The model under review builds one solid part; all positions refer to its coordinate system, in mm. Face numbers are marked on the shaded views. A direction names the side the tool comes from. Coordinates: 2 decimals unless noted, no trailing zeros. Order: outer loops, then holes, each group sorted by start corner. A loop starts at its lowest first (then second) coordinate and runs counter-clockwise, first axis right, second up. Notation, with made-up numbers: (86, 2.25) -> (116, 2.25) arc R12 ccw to (116, 6.25) -> close; hole circle Ø8 at (-15, 81). An arc over 180 degrees is marked (long way). Put each result on its own line as item: value.
from build123d import *

# Parameters (mm, degrees)
ESQUISSE2_W             = 60
ESQUISSE2_H             = 30
BOSS_EXTRU_1_DEPTH      = 15
ESQUISSE3_R             = 5
BOSS_EXTRU_2_DEPTH      = 6
BOSS_EXTRU_3_DEPTH      = 20
ESQUISSE5_R             = 5
ENL_V_MAT_EXTRU_1_DEPTH = 30
ESQUISSE6_W             = 3
ESQUISSE6_H             = 20
BOSS_EXTRU_4_DEPTH      = 15
CONG_2_R                = 10
CONG_3_R                = 10
CONG_4_R                = 10
CONG_5_R                = 10
ESQUISSE7_R             = 3
ENL_V_MAT_EXTRU_2_DEPTH = 27


with BuildPart() as part:
    # Esquisse2 → Boss.-Extru.1 (new body)
    with BuildSketch(Plane(origin=(0, 0, 0), x_dir=(1, 0, 0), z_dir=(0, 1, 0))):
        with Locations((-5, 0)):
            Rectangle(ESQUISSE2_W, ESQUISSE2_H)
    extrude(amount=BOSS_EXTRU_1_DEPTH)

    # Esquisse3 → Boss.-Extru.2 (add)
    with BuildSketch(Plane.XZ):
        with Locations(Location((-20, 0, 0), (0, 0, 90))):
            Circle(ESQUISSE3_R)
        with Locations(Location((20, 0, 0), (0, 0, 90))):
            Circle(ESQUISSE3_R)
    extrude(amount=BOSS_EXTRU_2_DEPTH)

    # Esquisse4 → Boss.-Extru.3 (add)
    with BuildSketch(Plane(origin=(0, 15, 0), x_dir=(1, 0, 0), z_dir=(0, 1, 0))):
        Polygon((-5, 15), (-15, 15), (-15, -15), (5, -15), (5, 15), align=None)
    extrude(amount=BOSS_EXTRU_3_DEPTH)

    # Esquisse5 → Enlèv. mat.-Extru.1 (cut)
    with BuildSketch(Plane(origin=(0, 0, -15), x_dir=(-1, 0, 0), z_dir=(0, 0, -1))):
        with Locations((5, 25)):
            Circle(ESQUISSE5_R)
    extrude(amount=-ENL_V_MAT_EXTRU_1_DEPTH, mode=Mode.SUBTRACT)

    # Esquisse6 → Boss.-Extru.4 (add)
    with BuildSketch(Plane.XY.offset(15)):
        with Locations((-13.5, 25)):
            Rectangle(ESQUISSE6_W, ESQUISSE6_H)
        with Locations((3.5, 25)):
            Rectangle(ESQUISSE6_W, ESQUISSE6_H)
    extrude(amount=BOSS_EXTRU_4_DEPTH)

    # Congé2
    cong_2_edges = [part.edges().sort_by_distance(p)[0] for p in [
        (3.5, 35, 30),
    ]]
    fillet(cong_2_edges, radius=CONG_2_R)

    # Congé3
    cong_3_edges = [part.edges().sort_by_distance(p)[0] for p in [
        (3.5, 15, 30),
    ]]
    fillet(cong_3_edges, radius=CONG_3_R - 0.0001)  # a hair under: the kernel refuses the full size

    # Congé4
    cong_4_edges = [part.edges().sort_by_distance(p)[0] for p in [
        (-13.5, 15, 30),
    ]]
    fillet(cong_4_edges, radius=CONG_4_R)

    # Congé5
    cong_5_edges = [part.edges().sort_by_distance(p)[0] for p in [
        (-13.5, 35, 30),
    ]]
    fillet(cong_5_edges, radius=CONG_5_R - 0.0001)  # a hair under: the kernel refuses the full size

    # Esquisse7 → Enlèv. mat.-Extru.2 (cut)
    with BuildSketch(Plane.ZY.offset(15)):
        with Locations((25, 25)):
            Circle(ESQUISSE7_R)
    extrude(amount=-ENL_V_MAT_EXTRU_2_DEPTH, mode=Mode.SUBTRACT)


solid = part.part
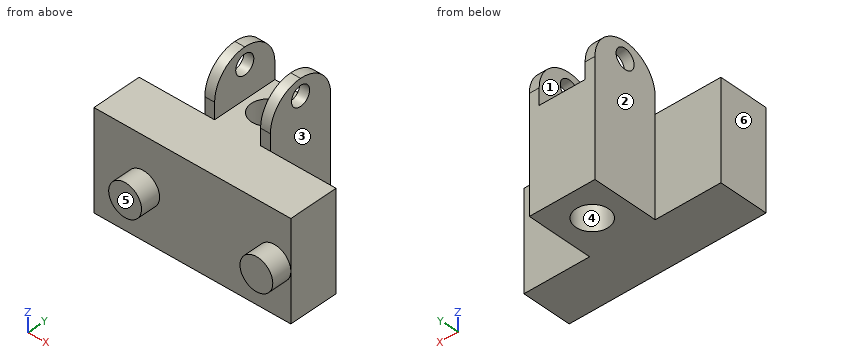
Item 1: Consider section C-C on z = 25. Write out the cut boundary in (x, y).
Answers below:
outline: (-15, 16.34) -> (-12, 16.34) -> (-12, 22) -> (-15, 22) -> close; (-15, 28) -> (-12, 28) -> (-12, 33.66) -> (-15, 33.66) -> close; (2, 16.34) -> (5, 16.34) -> (5, 22) -> (2, 22) -> close; (2, 28) -> (5, 28) -> (5, 33.66) -> (2, 33.66) -> close
Item 2: Consider section B-B on z = 8.5. Write out the cut boundary in (x, y).
Answers below:
outline: (-35, 0) -> (25, 0) -> (25, 15) -> (5, 15) -> (5, 35) -> (-15, 35) -> (-15, 15) -> (-35, 15) -> close; hole circle Ø10 at (-5, 25)
Item 3: For pin 1 Ø1 at (x, z) = (-8, -10.5) entering from -Y; pin 2 Ø4.5 at (y, z) = (23.5, 26) entering from -X; pin 3 Ø16 at (x, z) = (16.5, -6.5) entering from +Y; pin 4 Ø5 at (x, y) = (12.5, 19.5) entering from -Z, all flat-tipped, find the tip position at first contact; note any pin that passes through.
Answers below:
pin 1: y = 0
pin 2: x = -15
pin 3: y = 15
pin 4: through
Item 4: Consider section D-D on x = -20. Write out the cut boundary in (y, z), and give its area (3 significant figures).
Answers below:
outline: (-6, -5) -> (0, -5) -> (0, -15) -> (15, -15) -> (15, 15) -> (0, 15) -> (0, 5) -> (-6, 5) -> close
area: 510 mm^2
Item 5: For line 1 (Y direction, x = -5, z = -7); line 2 (X direction, y = 20.5, z = -0.5); line 3 (X direction, y = 26.5, z = 0), list the stretches that pass through material, from the lowest coordinate up. Write a range as from..to.
Answers below:
line 1: 0..20, 30..35
line 2: -15..-7.18, -2.82..5
line 3: -15..-9.77, -0.23..5
Item 6: For the marked faces 1, 2 and 3, list the 3-axis set-ups (+Z, -Z, +X, -X, +Y, -Y) from which the entire face can be reached by the end or side of a thin tool; tool diameter is ignored.
Answers below:
face 1: +Z, +Y, -Y
face 2: +Z, -Z, -X, +Y
face 3: +Z, -Z, +X, +Y
Item 7: Consider section A-A on x = -5. Write out the cut boundary in (y, z).
Answers below:
outline: (0, -15) -> (20, -15) -> (20, 15) -> (0, 15) -> close; (30, -15) -> (35, -15) -> (35, 15) -> (30, 15) -> close
Item 8: Mouldability with a two-part tool opening along X and no side actions: class the marked faces 4, 5 and 6 as +X half, -X half, draft (parallel to the pull), parting line (faces both ways), or undercut.
Answers below:
face 4: undercut
face 5: draft
face 6: -X half
